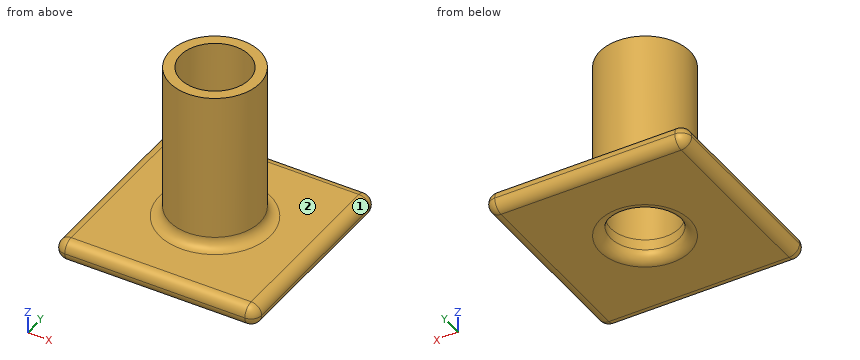
```python
from build123d import *

# Parameters (mm, degrees)
F0_R     = 8.5
F0_R_2   = 6.5
F1_DEPTH = 30
F2_W     = 38
F2_H     = 38
F2_R     = 6.5
F3_DEPTH = 4
F4_R     = 1.99999


# Not quite as in the source:
# - a fillet or chamfer is up to 0.001 mm smaller than in the source, because OpenCascade refuses the exact size


with BuildPart() as f1:
    # F0 (on Top) → F1 (new body)
    with BuildSketch(Plane.XY):
        Circle(F0_R)
        Circle(F0_R_2, mode=Mode.SUBTRACT)
    extrude(amount=F1_DEPTH)

    # F2 (on Top) → F3 (join)
    with BuildSketch(Plane.XY):
        Rectangle(F2_W, F2_H)
        Circle(F2_R, mode=Mode.SUBTRACT)
    extrude(amount=-F3_DEPTH)

    # F4 (radius 2 in the source; OpenCascade refuses exactly that, so slightly less here)
    f4_edges = [f1.edges().sort_by_distance(p)[0] for p in [
        (0, -19, -4),
        (19, 0, -4),
        (0, 19, -4),
        (-19, 0, -4),
        (-6.5, 0, -4),
        (0, -19, 0),
        (-19, 0, 0),
        (19, 0, 0),
        (0, 19, 0),
        (-8.5, 0, 0),
        (19, 19, -2),
        (-19, 19, -2),
        (19, -19, -2),
        (-19, -19, -2),
    ]]
    fillet(f4_edges, radius=F4_R)


solid = f1.part
```
Work out the finished part from the listing and answer in its coordinate system (mm). Face numbers are marked on the shaded views. A direction names the side the tool comes from. Give positions to 0.01 mm unless a question says otherwise; leave off trailing zeros. Order: outer loops, then holes, each group sorted by start corner. A loop starts at its lowest first (then second) coordinate and runs counter-clockwise, first axis right, second up. Notation, with made-up numbers: (45.5, 5.5) - (49.5, 5.5) arc R31 cw to (49.5, 32.5) - close; hole circle Ø7 at (28.5, -3). An arc over 180 degrees is marked (long way). One line per item, written item: value. Start each with the question number.
1. Consider line 1 (Z direction, x = -7, y = 15); line 2 (Y direction, x = 0, z = 11); line 3 (Y direction, x = 6, z = 14). Determine where each line is inside the solid, lowest interval first.
2. Which of the six approach directions +Z, -Z, +X, -X, +Y, -Y give full straight-line access (tool end or side, diameter ignored) to the marked faces 1 and 2?
3. Section D-D, the plane z = 20.5 is taken. Write down the section's boundary in (x, y).
4. Each of these flat-tipped pins is pushed along its axis until it touches: pin 1 Ø17 at (x, y) = (0, 0) entering from +Z; pin 2 Ø1.5 at (x, z) = (10.5, 11.5) entering from -Y; pin 3 Ø3 at (y, z) = (-6, 16.5) entering from +X; pin 4 Ø12 at (x, z) = (-13.5, 17) entering from -Y. Where does it stop, or does it pass through?
Filled sheet:
1. line 1: -4 to 0
1. line 2: -8.5 to -6.5, 6.5 to 8.5
1. line 3: -6.02 to -2.5, 2.5 to 6.02
2. face 1: +Z, +X, +Y, -Y
2. face 2: +Z
3. outline: circle Ø17 at (0, 0); hole circle Ø13 at (0, 0)
4. pin 1: z = 30
4. pin 2: through
4. pin 3: x = 7.21
4. pin 4: y = -4
